Geometry check sheet. Reference: the model listing, model coordinates, mm. Coordinates: 2 decimals unless noted, no trailing zeros. Order: outer loops, then holes, each group sorted by start corner. A loop starts at its lowest first (then second) coordinate and runs counter-clockwise, first axis right, second up. Notation, with made-up numbers: M 10,-26 L 53,-26 A23 ccw 53,11 Z; hole C 39,67 d6. An arc over 180 degrees is marked long. One line per item, written item: value. Start each with the question number.
1) Sectioned sample at D-D, the plane x = -61. Enter the section's corners in (y, z), then the cut area to 3 significant figures.
2) Thickness scan on L1, parallel to X at y = -5.5, z = 3; L2, parallel to Z at x = -44, y = -11.75; L3, parallel to X at y = -1, z = 7. Record the ranges inside material, lowest first. Write a range as from..to.
3) Draft check along Z on faces 1 (the cylindrical face through (-53.054, -6.439, 11.059)), 2 (the flat face through (-28, -6, 29.314)), 3 (the flat face through (-28, 0, -9)), 4 (the cylindrical face through (-9.747, -6.261, -43.483)). Enter one of: pulls with the +Z half, pulls with the -Z half, needs draft (parallel to the pull), parting line crosses it, or undercut.
4) Sectioned sample at A-A, the plane y = -4.75. Enter the section's corners in (x, z) (3 decimals), then the cut area to 3 significant figures.
5) Sectioned sample at B-B, the plane x = -51. Enter the section's corners in (y, z).
6) Sectioned sample at C-C, the plane z = -38. Enter the section's corners in (x, y).
7) Go/stop test with flat-tipped pins: P1, Ø4, axis at y = -4, z = 12, coming from the +X side; P2, Ø1, axis at y = -6, z = 14.5, coming from the -X side; P3, Ø2, axis at y = -2, z = -35.5, coming from the +X side. Record where each tip stops, or that it passes through.
```python
from build123d import *

# Parameters (mm, degrees)
F1_DEPTH = 12.7
F3_D     = 6.35
F4_SIZE  = 5.08


with BuildPart() as f1:
    # F0 (on Front) → F1 (new body)
    with BuildSketch(Plane.XZ):
        with BuildLine():
            ThreePointArc((-43.925832, 29.31416), (-61.886345, 21.874673), (-69.325832, 3.91416))
            Line((-69.325832, 3.91416), (-69.325832, -47.419965))
            Line((-69.325832, -47.419965), (-23.331021, -47.419965))
            ThreePointArc((-23.331021, -47.419965), (-9.575842, -43.37307), (-0.203796, -32.521939))
            Line((-0.203796, -32.521939), (11.572779, -6.587813))
            ThreePointArc((11.572779, -6.587813), (9.798658, 17.669339), (-11.554446, 29.31416))
            Line((-11.554446, 29.31416), (-43.925832, 29.31416))
        make_face()
    extrude(amount=F1_DEPTH)

    # F3 (through all)
    with Locations(Plane(origin=(0, 0, 0), x_dir=(-1, 0, 0), z_dir=(0, 1, 0))):
        with Locations((50.714333, 8.912938)):
            Hole(F3_D / 2)

    # F4
    f4_edges = [f1.edges().sort_by_distance(p)[0] for p in [
        (-69.325832, -6.35, -47.419965),
    ]]
    chamfer(f4_edges, length=F4_SIZE)


solid = f1.part
```
Final values:
1. outline: M -12.7,-47.42 L 0,-47.42 L 0,22.72 L -12.7,22.72 Z
1. area: 891 mm^2
2. L1: x = -69.33..13.83
2. L2: z = -47.42..29.31
2. L3: x = -69.14..-53.25, -48.18..13.66
3. face 1: undercut
3. face 2: pulls with the +Z half
3. face 3: needs draft
3. face 4: pulls with the -Z half
4. outline: M -69.326,-42.34 L -64.246,-47.42 L -23.331,-47.42 A25.4 ccw -0.204,-32.522 L 11.573,-6.588 A25.4 ccw -11.554,29.314 L -43.926,29.314 A25.4 ccw -69.326,3.914 Z; hole C -50.714,8.913 d6.35
4. area: 5,540 mm^2
5. outline: M -12.7,-47.42 L 0,-47.42 L 0,5.75 L -12.7,5.75 Z; M -12.7,12.08 L 0,12.08 L 0,28.31 L -12.7,28.31 Z
6. outline: M -69.33,-12.7 L -3.59,-12.7 L -3.59,0 L -69.33,0 Z
7. P1: stops at x = 13.11
7. P2: stops at x = -67.24
7. P3: stops at x = -1.21
